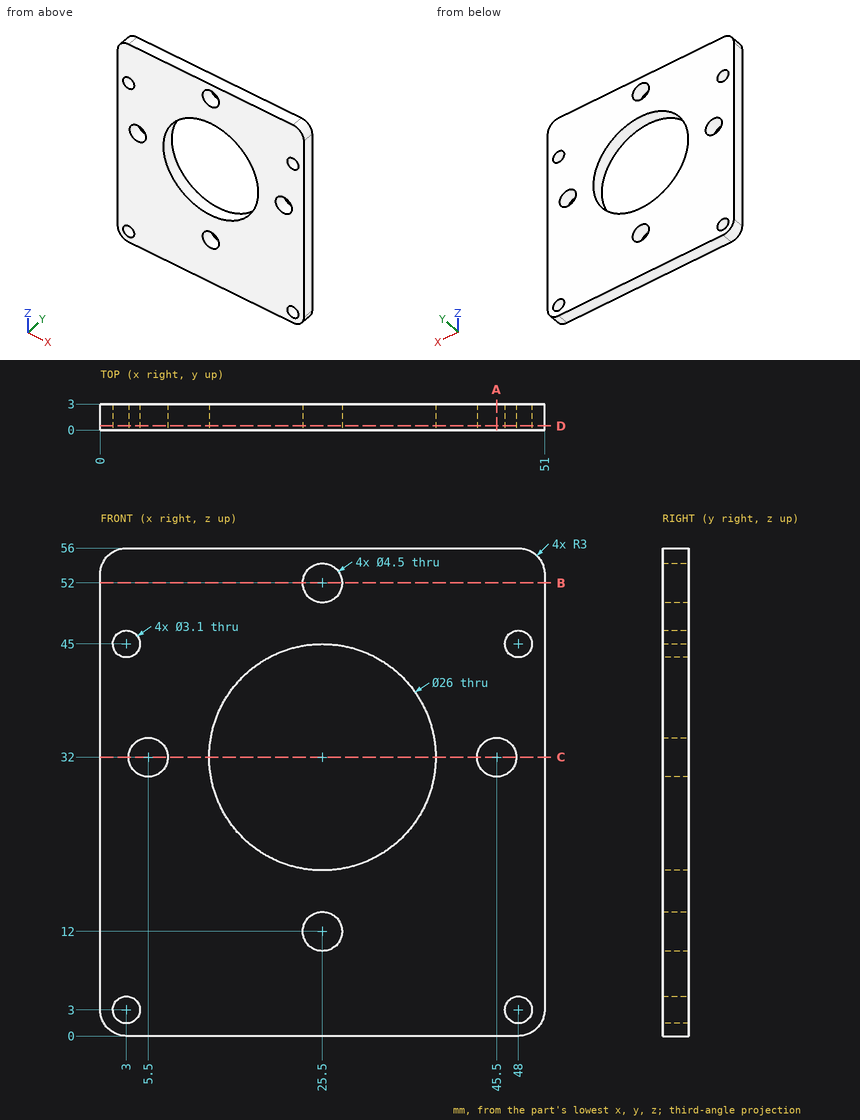
Geometry: see drawing. Coordinates: mm, zero at the bounding-box minimum. Coordinates: 2 decimals unless noted, no trailing zeros. Loops run counter-clockwise (first coordinate to the right, second up) from the corner with the lowest first, then second, coordinate; pieces in that order, holes last. Notation, with made-up numbers: (-36.5, 19) -> (-18.5, 19) arc R21 cw to (-18.5, 41) -> close; hole circle Ø4 at (67.25, -5). An arc over 180 degrees is marked (long way). Write item = value, one per line. Start each with the question number.
Item 1: First-contact query: P1, Ø2.5, axis at x = 3, z = 45, coming from the +Y side. Flat tip, straight axial feed; report the tip coordinate or a pass-through.
Item 2: Cut plane B-B, the plane z = 52. Return loops of the section in (x, y), plus the area to 4 significant figures.
Item 3: Cut plane A-A, the plane x = 45.5. Return loops of the section in (y, z).
Item 4: Cut plane C-C, the plane z = 32. Return loops of the section in (x, y).
Item 5: Cut plane D-D, the plane y = 0.5. Count the separate pieces of the cut face and the enclosed holes in it, plus the area to 3 significant figures.
Item 6: Material intervals for line 1 (X direction, y = 2.8, z = 12); line 2 (X direction, y = 1.95, z = 4); line 3 (Z direction, x = 26, y = 0.65), sorted ascending.
Ans:
q1.P1 = through
q2.outline = (0, 0) -> (23.25, 0) -> (23.25, 3) -> (0, 3) -> close; (27.75, 0) -> (51, 0) -> (51, 3) -> (27.75, 3) -> close
q2.area = 139.5 mm²
q3.outline = (0, 0) -> (3, 0) -> (3, 29.75) -> (0, 29.75) -> close; (0, 34.25) -> (3, 34.25) -> (3, 56) -> (0, 56) -> close
q4.outline = (0, 0) -> (3.25, 0) -> (3.25, 3) -> (0, 3) -> close; (7.75, 0) -> (12.5, 0) -> (12.5, 3) -> (7.75, 3) -> close; (38.5, 0) -> (43.25, 0) -> (43.25, 3) -> (38.5, 3) -> close; (47.75, 0) -> (51, 0) -> (51, 3) -> (47.75, 3) -> close
q5.separate_pieces = 1
q5.enclosed_holes = 9
q5.area = 2,220 mm²
q6.line_1 = 0 to 23.25, 27.75 to 51
q6.line_2 = 0 to 1.82, 4.18 to 46.82, 49.18 to 51
q6.line_3 = 0 to 9.81, 14.19 to 19.01, 44.99 to 49.81, 54.19 to 56
